The listing builds one solid part. Answer for the finished solid, in the listing's coordinates (mm). Face numbers are marked on the shaded views. A direction names the side the tool comes from. Give positions to 0.01 mm unless a question says otherwise; leave off trailing zeros. Loops run counter-clockwise (first coordinate to the right, second up) from the corner with the lowest first, then second, coordinate; pieces in that order, holes last. Notation, with made-up numbers: (-14.5, 80.25) - (25.5, 80.25) arc R23 cw to (25.5, 113.25) - close; hole circle Ø8 at (-21.5, 1). An arc over 180 degrees is marked (long way). Write each question's results on one line, items separated by ' | '.
Autodesk Inventor part; units mm, degrees
ref_plane "YZ Plane" through (0, 0, 0) normal (1, 0, 0) x (0, 1, 0)
ref_plane "XZ Plane" through (0, 0, 0) normal (0, 1, 0) x (-1, 0, 0)
ref_plane "XY Plane" through (0, 0, 0) normal (0, 0, 1) x (1, 0, 0)
sketch "Bottom" plane through (0, 0, 0) normal (0, 1, 0) x (-1, 0, 0)
  line L0 (-10.675, -10.675) -> (82.525, -10.675)
  line L1 (82.525, -10.675) -> (82.525, 10.675)
  line L2 (82.525, 10.675) -> (-10.675, 10.675)
  line L3 (-10.675, 10.675) -> (-10.675, -10.675) construction
  line L4 (-10.675, 1.5) -> (8.35, 1.5)
  line L5 (8.35, 1.5) -> (8.35, -1.5)
  line L6 (8.35, -1.5) -> (-10.675, -1.5)
  line L7 (-10.675, 1.5) -> (-10.675, 10.675)
  line L8 (-10.675, -1.5) -> (-10.675, -10.675)
  circle A0 centre (71.85, 0) radius 5.3375
  point P0 (0, 0)
  point P1 (8.35, 0)
  dimension "Width" = 21.35
  dimension "d2" = 10.675
  dimension "d3" = 93.2
  dimension "d4" = 10.675
  dimension "d8" = 9.175
  dimension "d9" = 9.175
  dimension "d10" = 3
  dimension "ArmMount" = 19.025
  dimension "d15" = 19.025
  dimension "d16" = 10.675
  dimension "d19" = 10.675
  dimension "d22" = 10.675
  dimension "d23" = 10.675
extrude "Extrusion1" add sketch "Bottom" along normal blind 19.35 contours L8 L6 L5 L4 L7 L2 L1 L0 | A0
extrude "Extrusion2" add sketch "Bottom" along normal blind 48.375 contours A0
hole "Hole1" at (-8.35, 0, 0) direction (0, 1, 0) diameter 5.5 end through all
sketch "Side" plane through (10.675, 0, -10.675) normal (0, 0, -1) x (-1, 0, 0)
  line L0 (0, 19.35) -> (93.2, 19.35)
  line L1 (0, 0) -> (0, 19.35)
  line L2 (8.1375, 2.1694) -> (1.6375, 5.9222)
  line L3 (1.6375, 5.9222) -> (1.6375, 13.4278)
  line L4 (1.6375, 13.4278) -> (8.1375, 17.1806)
  line L5 (8.1375, 17.1806) -> (14.6375, 13.4278)
  line L6 (14.6375, 13.4278) -> (14.6375, 5.9222)
  line L7 (14.6375, 5.9222) -> (8.1375, 2.1694)
  point P0 (10.675, 0)
  point P1 (8.1375, 9.675)
  point P2 (8.1375, 9.675)
  dimension "d31" = 9.675
  dimension "d32" = 8.1375
  dimension "Nut" = 6.5
  dimension "d44" = 2.1694
hole "Hole2" at (2.5375, 9.675, -10.675) direction (0, 0, 1) diameter 6.35 end through all
extrude "Extrusion3" cut sketch "Side" against normal blind 4.5875
fillet "Fillet1" radius 10.675 2 edges at (-82.525, 9.675, -10.675) (-82.525, 9.675, 10.675)
fillet "Fillet2" radius 4 1 edges at (-66.5125, 48.375, 0)
fillet "Fillet3" radius 4.8 1 edges at (-66.5125, 19.35, 0)
equation "\"d9\" = d8"
equation "\"d19\" = d2"
equation "\"d22\" = d2"
equation "\"d23\" = d2"
equation "\"d20\" = 2.5 * Thickness"
equation "\"d45\" = 0.5 * d9"
equation "\"d47\" = 0.5 * Width"
properties part number "Egg_Turner_Motor_Arm"
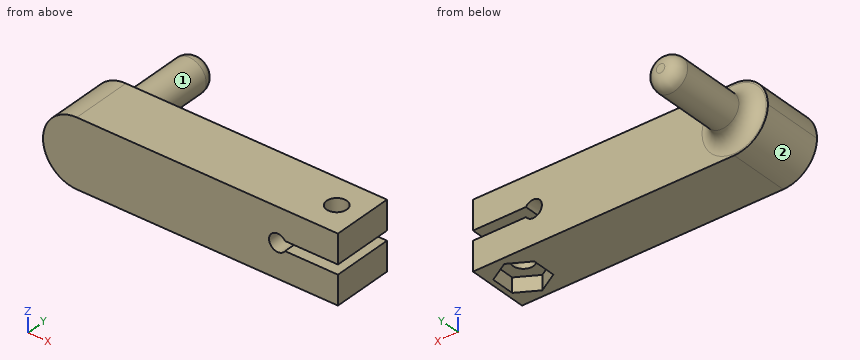
Item 1: A cutting plane is placed at B-B, the plane y = 22.5. Determine the outline of the cut face in (x, z).
Values found:
outline: circle Ø11.26 at (-71.85, 0)
Item 2: A cutting plane is placed at C-C, the plane x = -35. Determine the outline of the cut face in (y, z) (3 decimals), plus the area to 3 significant figures.
Values found:
outline: (0, -10.675) - (19.35, -10.675) - (19.35, 10.675) - (0, 10.675) - close | area: 413 mm²
Item 3: For the marked faces 1 and 2, determine the directions among +Z, -Z, +X, -X, +Y, -Y from which every point of the face is accessible in a straight line to the end or side of a thin tool.
Values found:
face 1: +Y | face 2: -Z, -X, +Y, -Y
Item 4: Find the intervals of material crossed by line 1 along Y through (x, z) = (-40, 9.5); line 2 along X through (y, z) = (8, -5.5) (3 decimals); line 3 along Y through (x, z) = (3.5, -8.75), in increasing order. Write a range as [from, to].
Values found:
line 1: y = [0, 19.35] | line 2: x = [-80.999, -0.16], [5.235, 10.675] | line 3: y = [0, 2.73], [16.62, 19.35]
Item 5: A cutting plane is placed at A-A, the plane x = -8.35. Determine the outline of the cut face in (y, z) (3 decimals).
Values found:
outline: (0, -10.675) - (19.35, -10.675) - (19.35, -2.75) - (0, -2.75) - close; (0, 2.75) - (19.35, 2.75) - (19.35, 10.675) - (0, 10.675) - close
Item 6: Flat-ended cylindrical pins translate along their axes: P1, Ø7.5, axis at x = 2.54, y = 9.68, coming from the +Z side (3 decimals); P2, Ø5, axis at x = 1.5, y = 7, coming from the -Z side; P3, Ø5, axis at y = 11, z = -7.5, coming from the -X side; P4, Ø1.5, axis at y = 6.5, z = -6.5, coming from the -X side. Find the tip coordinate at first contact, or state that the pin passes through.
Values found:
P1: stops at z = 10.675 | P2: stops at z = -6.09 | P3: stops at x = -81.28 | P4: stops at x = -80.84
